The listing builds one solid part. Answer for the finished solid, in the listing's coordinates (mm). Face numbers are marked on the shaded views. A direction names the side the tool comes from. Round coordinates to 2 decimals unless told otherwise and drop trailing zeros. Write each loop counter-clockwise with the first axis right and the second up, starting at its lowest first coordinate (ties: lowest second). Pieces come first, ordered by that corner, then holes.
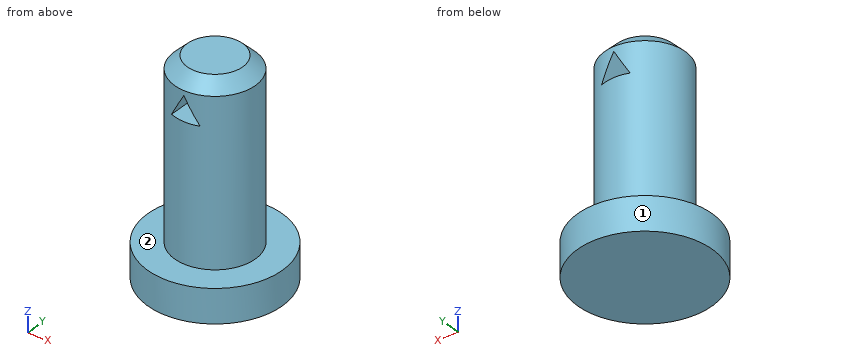
from build123d import *

# Parameters (mm, degrees)
F0_R     = 4
F1_DEPTH = 2
F2_R     = 2.4
F3_DEPTH = 10.5
F5_DEPTH = 5
F6_SIZE  = 0.75


with BuildPart() as f1:
    # F0 (on Top) → F1 (new body)
    with BuildSketch(Plane.XY):
        Circle(F0_R)
    extrude(amount=F1_DEPTH)

    # F2 (on face) → F3 (join)
    with BuildSketch(Plane.XY.offset(2)):
        Circle(F2_R)
    extrude(amount=F3_DEPTH)

    # F4 (on Front) → F5 (cut, symmetric)
    with BuildSketch(Plane.XZ):
        Polygon((0, 11.472243), (-0.85, 10), (0.85, 10), align=None)
    extrude(amount=F5_DEPTH, both=True, mode=Mode.SUBTRACT)

    # F6
    f6_edges = [f1.edges().sort_by_distance(p)[0] for p in [
        (-2.4, 0, 12.5),
    ]]
    chamfer(f6_edges, length=F6_SIZE)


solid = f1.part
1. A tool of negligible diameter and unlimited length cuts with its end or side. For the marked faces 1 and 2, from which of +Z, -Z, +X, -X, +Y, -Y can it reach the whole face along a straight path? Write none if from no direction.
Geometry says:
face 1: +Z, -Z
face 2: +Z
2. Section A-A on z = 10.5 is taken. Determine the outline of the cut face in (x, y).
Geometry says:
outline: (-0.56, -2.33) - (-0.56, 2.33) arc R2.4 ccw to start; (0.56, -2.33) arc R2.4 ccw to (0.56, 2.33) - close
3. Section B-B on z = 1.5 is taken. Determine the outline of the cut face in (x, y).
Geometry says:
outline: circle Ø8 at (0, 0)
4. Section C-C on y = 3 is taken. Determine the outline of the cut face in (x, z).
Geometry says:
outline: (-2.65, 0) - (2.65, 0) - (2.65, 2) - (-2.65, 2) - close
5. Given pin 1 (3 mm diameter, centred on x = 0.5, z = 4.5, fed in from -Y); pin 2 (1.5 mm diameter, centred on x = -1.5, y = 1, fed in from +Z); pin 3 (2 mm diameter, centred on y = -2.5, z = 3.5, fed in from -X); pin 4 (4 mm diameter, centred on x = 0.5, z = 10, fed in from +Y), each flat-ended and moving along its own axis, determine where each tip first touches the part or whether it passes through.
Geometry says:
pin 1: stops at y = -2.4
pin 2: stops at z = 12.5
pin 3: stops at x = -1.87
pin 4: stops at y = 2.4
6. Straight lines are drawn through the part: line 1 along Z through (x, y) = (3, -2.5); line 2 along Y through (x, z) = (0, 9); line 3 along Z through (x, y) = (-0.75, 1). For each, find the intervals that lie inside material, in ascending order.
Geometry says:
line 1: z = 0 to 2
line 2: y = -2.4 to 2.4
line 3: z = 0 to 10, 10.17 to 12.5
